```python
from build123d import *

# Parameters (mm, degrees)
F1_DEPTH = 6.35
F2_W     = 2.2056519679
F2_H     = 1.4280619276
F2_H_2   = 2.76814439
F2_W_2   = 1.6606743359
F2_W_3   = 1.7216736962
F2_H_3   = 2.0531332773
F3_DEPTH = 25.4
F4_R     = 2.4226901475
F4_R_2   = 2.1898139235
F4_R_3   = 2.1544927731
F5_DEPTH = 25.4
F7_DEPTH = 25.4
F8_W     = 0.762
F8_H     = 0.8323322826
F8_H_2   = 0.6916765124
F8_W_2   = 1.2084901007
F9_DEPTH = 25.4


with BuildPart() as f1:
    # F0 (on Front) → F1 (new body)
    with BuildSketch(Plane.XZ):
        with BuildLine():
            Line((-8.1283105537, 28.4980535507), (-8.1283105537, 0))
            Line((-8.1283105537, 0), (0, -18.5090452433))
            Line((0, -18.5090452433), (0, 0))
            Line((0, 0), (0, 28.302192688))
            ThreePointArc((0, 28.302192688), (-3.9685561641, 32.3675276661), (-8.1283105537, 28.4980535507))
        make_face()
        with BuildLine():
            Line((0, 0), (0, -18.5090452433))
            Line((0, -18.5090452433), (16.5504161268, -18.5090452433))
            ThreePointArc((16.5504161268, -18.5090452433), (19.4883598015, -15.5711015686), (16.5504161268, -12.633157894))
            Line((16.5504161268, -12.633157894), (4.2110523209, -12.633157894))
            Line((4.2110523209, -12.633157894), (0, 0))
        make_face()
    extrude(amount=F1_DEPTH)

    # F2 (on Front) → F3 (cut)
    with BuildSketch(Plane.XZ):
        with Locations((-4.1150925963, 24.9122383648)):
            Rectangle(F2_W, F2_H)
        with Locations((-4.1150925963, 27.0103415236)):
            Rectangle(F2_W, F2_H_2)
        with Locations((-2.1819294444, 27.0103415236)):
            Rectangle(F2_W_2, F2_H_2)
        with Locations((-6.0787554284, 27.0103415236)):
            Rectangle(F2_W_3, F2_H_2)
        with Locations((-4.1150925963, 29.4209803573)):
            Rectangle(F2_W, F2_H_3)
    extrude(amount=F3_DEPTH, mode=Mode.SUBTRACT)

    # F4 (on Front) → F5 (cut)
    with BuildSketch(Plane.XZ):
        with Locations((-4.1131214239, 20.8593998104)):
            Circle(F4_R)
        with Locations((-3.9172577672, 14.9835133925)):
            Circle(F4_R)
        with Locations((-3.9172577672, 8.9117623866)):
            Circle(F4_R)
        with Locations((-3.7213957403, 2.4482863955)):
            Circle(F4_R)
        with Locations((-3.5255320836, -3.2317379955)):
            Circle(F4_R)
        with Locations((2.154491609, -14.5917870104)):
            Circle(F4_R_2)
        with Locations((8.030379191, -14.9835133925)):
            Circle(F4_R_2)
        with Locations((12.9269538447, -14.9835133925)):
            Circle(F4_R_3)
    extrude(amount=F5_DEPTH, mode=Mode.SUBTRACT)

    # F6 (on Front) → F7 (cut)
    with BuildSketch(Plane.XZ):
        with BuildLine():
            ThreePointArc((0, -6.3673276454), (-2.0752432977, -5.6200849272), (-3.2373126596, -7.4948119))
            Line((-3.2373126596, -7.4948119), (-1.0640458204, -12.2008332983))
            ThreePointArc((-1.0640458204, -12.2008332983), (0.9608741924, -12.3759405779), (1.7464946723, -10.5014368892))
            Line((1.7464946723, -10.5014368892), (0, -6.3673276454))
        make_face()
    extrude(amount=F7_DEPTH, mode=Mode.SUBTRACT)

    # F8 (on Front) → F9 (cut)
    with BuildSketch(Plane.XZ):
        with Locations((17.1117875725, -16.1442225721)):
            Rectangle(F8_W, F8_H)
        with Locations((17.1117875725, -15.3822181746)):
            Rectangle(F8_W, F8_H_2)
        with Locations((18.0970326229, -15.3822181746)):
            Rectangle(F8_W_2, F8_H_2)
        with Locations((16.1265425221, -15.3822181746)):
            Rectangle(F8_W_2, F8_H_2)
        with Locations((17.1117875725, -14.6202137772)):
            Rectangle(F8_W, F8_H)
    extrude(amount=F9_DEPTH, mode=Mode.SUBTRACT)


solid = f1.part
```
Read the model definition and answer for the solid it produces. Units are mm, in the model's axes. A direction names the side the tool comes from. Round coordinates to 2 decimals unless told otherwise and drop trailing zeros. Write each loop counter-clockwise with the first axis right and the second up, starting at its lowest first coordinate (ties: lowest second). Pieces come first, ordered by that corner, then holes. Notation, with made-up numbers: (-32, -37.75) - (-5, -37.75) arc R21 cw to (-5, -5.75) - close; hole circle Ø9 at (23.5, 2.25). An arc over 180 degrees is marked (long way). One line per item, written item: value.
Q1. For a pull along Z with two mould halves and no side action, classify faces 1 (the flat face through (8, -3, -18.509)), 2 (the flat face through (-5.218, -3, 25)), 3 (the flat face through (0, -3, 14)) as pulls with the +Z half, pulls with the -Z half, needs draft (parallel to the pull), parting line crosses it, or undercut.
The answers:
face 1: pulls with the -Z half
face 2: undercut
face 3: needs draft
Q2. Find section C-C (z = 26.5). Determine the outline of the cut face in (x, y).
The answers:
outline: (-8.13, -6.35) - (-6.94, -6.35) - (-6.94, 0) - (-8.13, 0) - close; (-1.35, -6.35) - (0, -6.35) - (0, 0) - (-1.35, 0) - close
Q3. Find section D-D (x = 1.25). Determine the outline of the cut face in (y, z).
The answers:
outline: (-6.35, -18.51) - (0, -18.51) - (0, -16.59) - (-6.35, -16.59) - close; (-6.35, -12.6) - (0, -12.6) - (0, -12.16) - (-6.35, -12.16) - close; (-6.35, -9.33) - (0, -9.33) - (0, -3.75) - (-6.35, -3.75) - close
Q4. Find section B-B (z = -13.5). Determine the outline of the cut face in (x, y), and give its area (3 significant figures).
The answers:
outline: (-2.2, -6.35) - (0.26, -6.35) - (0.26, 0) - (-2.2, 0) - close; (4.05, -6.35) - (6.42, -6.35) - (6.42, 0) - (4.05, 0) - close; (9.64, -6.35) - (11.36, -6.35) - (11.36, 0) - (9.64, 0) - close; (14.49, -6.35) - (18.63, -6.35) - (18.63, 0) - (14.49, 0) - close
area: 67.9 mm2
Q5. Each of these flat-tipped pins is pushed along its axis until it touches: P1, Ø0.8, axis at y = -4.5, z = -15, coming from the +X side; P2, Ø0.8, axis at y = -2, z = -15.5, coming from the -X side; P3, Ø1.3, axis at x = 16.5, y = -3, coming from the +Z side; P4, Ø3, axis at x = -3.92, z = 14.98, coming from the -Y side. Where does it stop, or does it pass through?
The answers:
P1: stops at x = 19.48
P2: stops at x = -1.5
P3: stops at z = -12.63
P4: passes through
Q6. Which of the six approach directions +Z, -Z, +X, -X, +Y, -Y give full straight-line access (tool end or side, diameter ignored) to faces 4 (the cylindrical face through (-2.04, -3.13, -5.61)), 5 (the flat face through (2, -3, -6))?
The answers:
face 4: +Y, -Y
face 5: +Z, +X, +Y, -Y
Q7. Straight lines are drawn through the part: line 1 (Z direction, x = 15.75, y = -5.5); line 2 (X direction, y = -1.5, z = 15); line 3 (X direction, y = -5, z = 5). For each, find the intervals that lie inside material, in ascending order. Write a range as from..to.
The answers:
line 1: z = -18.51..-15.73, -15.04..-12.63
line 2: x = -8.13..-6.34, -1.49..0
line 3: x = -8.13..0
Q8. Find section A-A (x = 13). Determine the outline of the cut face in (y, z).
The answers:
outline: (-6.35, -18.51) - (0, -18.51) - (0, -17.14) - (-6.35, -17.14) - close; (-6.35, -12.83) - (0, -12.83) - (0, -12.63) - (-6.35, -12.63) - close
